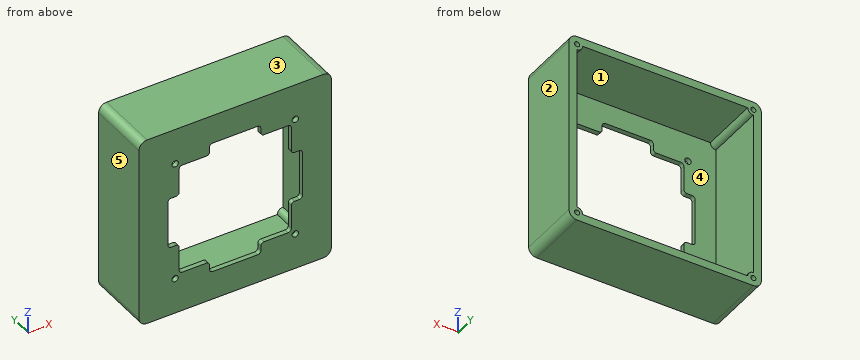
Autodesk Inventor part; units mm, degrees
ref_plane "YZ Plane" through (0, 0, 0) normal (1, 0, 0) x (0, 1, 0)
ref_plane "XZ Plane" through (0, 0, 0) normal (0, 1, 0) x (-1, 0, 0)
ref_plane "XY Plane" through (0, 0, 0) normal (0, 0, 1) x (1, 0, 0)
sketch "Sketch1" plane through (0, 0, 0) normal (0, 1, 0) x (-1, 0, 0)
  line L0 (-55, 55) -> (55, 55)
  line L1 (55, 55) -> (55, -55)
  line L2 (55, -55) -> (-55, -55)
  line L3 (-55, -55) -> (-55, 55)
  line L4 (-55, 55) -> (55, -55) construction
  line L5 (55, 55) -> (-55, -55) construction
  line L6 (-12.5, 37.5) -> (12.5, 37.5) construction
  line L7 (12.5, 37.5) -> (12.5, -37.5) construction
  line L8 (12.5, -37.5) -> (-12.5, -37.5) construction
  line L9 (-12.5, -37.5) -> (-12.5, 37.5) construction
  line L10 (-12.5, 37.5) -> (12.5, -37.5) construction
  line L11 (12.5, 37.5) -> (-12.5, -37.5) construction
  line L12 (-37.5, 37.5) -> (37.5, 37.5) construction
  line L13 (37.5, 37.5) -> (37.5, -37.5) construction
  line L14 (37.5, -37.5) -> (-37.5, -37.5) construction
  line L15 (-37.5, -37.5) -> (-37.5, 37.5)
  line L16 (-37.5, 37.5) -> (37.5, -37.5) construction
  line L17 (37.5, 37.5) -> (-37.5, -37.5) construction
  circle A0 centre (37.5, -37.5) radius 2
  circle A1 centre (37.5, 37.5) radius 2
  circle A2 centre (-37.5, 37.5) radius 2
  circle A3 centre (-37.5, -37.5) radius 2
  point P0 (0, 0)
  dimension "d0" = 110
  dimension "d1" = 110
  dimension "d2" = 25
  dimension "d3" = 75
  dimension "d4" = 75
  dimension "d5" = 4
  dimension "d6" = 4
  dimension "d7" = 4
  dimension "d8" = 4
extrude "Extrusion1" add sketch "Sketch1" along normal blind 3
sketch "Sketch3" plane through (0, 3, 0) normal (0, 1, 0) x (1, 0, 0)
  line L0 (35, -35) -> (-35, -35)
  line L1 (-35, -35) -> (-35, 35)
  line L2 (-35, 35) -> (35, 35)
  line L3 (35, 35) -> (35, -35)
  line L4 (35, -35) -> (-35, 35) construction
  line L5 (-35, -35) -> (35, 35) construction
  point P0 (0, 0)
  dimension "d18" = 70
  dimension "d19" = 70
extrude "Extrusion3" cut sketch "Sketch3" against normal blind 3
fillet "Fillet1" radius 2 4 edges at (-35, 1.5, 35) (-35, 1.5, -35) (35, 1.5, -35) (35, 1.5, 35)
sketch "Sketch4" plane through (0, 3, 0) normal (0, 1, 0) x (1, 0, 0)
  line L0 (28, -16) -> (42, -16)
  line L1 (42, -16) -> (42, 16)
  line L2 (42, 16) -> (28, 16)
  line L3 (28, 16) -> (28, -16)
  line L4 (28, -16) -> (42, 16) construction
  line L5 (42, -16) -> (28, 16) construction
  line L6 (35, 33) -> (35, -33)
  point P0 (0, 0)
  point P1 (35, 0)
  dimension "d23" = 14
  dimension "d24" = 32
extrude "Extrusion4" cut sketch "Sketch4" against normal blind 3
pattern_circular "Circular Pattern2" count 4 over 360 about axis through (0, 0, 0) along (0, 1, 0) of "Extrusion4"
fillet "Fillet2" radius 2 16 edges at (16, 1.5, 35) (-16, 1.5, 35) (16, 1.5, 42) (-16, 1.5, 42) (-35, 1.5, 16) (-42, 1.5, 16) (-42, 1.5, -16) (-35, 1.5, -16) (-16, 1.5, -35) (-16, 1.5, -42) (16, 1.5, -42) (16, 1.5, -35) (35, 1.5, -16) (42, 1.5, -16) (42, 1.5, 16) (35, 1.5, 16)
sketch "Sketch5" plane through (0, 0, 0) normal (0, -1, 0) x (1, 0, 0)
  line L0 (55, -55) -> (-55, -55)
  line L1 (-55, 55) -> (55, 55)
  line L2 (55, 55) -> (55, -55)
  line L3 (55, -55) -> (-55, -55)
  line L4 (-55, -55) -> (-55, 55)
  line L5 (-55, 55) -> (55, -55) construction
  line L6 (55, 55) -> (-55, -55) construction
  line L7 (-60, 60) -> (60, 60)
  line L8 (60, 60) -> (60, -60)
  line L9 (60, -60) -> (-60, -60)
  line L10 (-60, -60) -> (-60, 60)
  line L11 (-60, 60) -> (60, -60) construction
  line L12 (60, 60) -> (-60, -60) construction
  point P0 (0, 0)
  dimension "d31" = 5
extrude "Extrusion5" add sketch "Sketch5" against normal blind 40
sketch "Sketch6" plane through (0, 40, 0) normal (0, 1, 0) x (1, 0, 0)
  line L0 (-55, -55) -> (55, -55)
  circle A0 centre (-55, -55) radius 3.5
  line L1 (-55, -55) -> (-55, 55)
  circle A1 centre (-55, 55) radius 3.5
  line L2 (55, 55) -> (55, -55)
  circle A2 centre (55, 55) radius 3.5
  circle A3 centre (55, -55) radius 3.5
  point P0 (0, 0)
  dimension "d34" = 7
  dimension "d35" = 7
  dimension "d36" = 7
  dimension "d37" = 7
extrude "Extrusion6" add sketch "Sketch6" against normal up to surface (37 mm away)
sketch "Sketch7" plane through (0, 40, 0) normal (0, 1, 0) x (1, 0, 0)
  arc A0 (55, -51.5) -> (51.5, -55) centre (55, -55) ccw
  circle A1 centre (55, -55) radius 1.6
  arc A2 (51.5, 55) -> (55, 51.5) centre (55, 55) ccw
  circle A3 centre (55, 55) radius 1.6
  arc A4 (-55, 51.5) -> (-51.5, 55) centre (-55, 55) ccw
  circle A5 centre (-55, 55) radius 1.6
  arc A6 (-51.5, -55) -> (-55, -51.5) centre (-55, -55) ccw
  circle A7 centre (-55, -55) radius 1.6
  point P0 (0, 0)
  dimension "d40" = 3.2
  dimension "d41" = 3.2
  dimension "d42" = 3.2
  dimension "d43" = 3.2
extrude "Extrusion7" cut sketch "Sketch7" against normal blind 4.5
fillet "Fillet3" radius 5 4 edges at (60, 20, -60) (-60, 20, -60) (60, 20, 60) (-60, 20, 60)
properties part number "3D printed box"
Design review of the part built by this model. Coordinates are the model's own, in mm. Face numbers are marked on the shaded views. A direction names the side the tool comes from. Round coordinates to 2 decimals unless told otherwise and drop trailing zeros. Loops run counter-clockwise (first coordinate to the right, second up) from the corner with the lowest first, then second, coordinate; pieces in that order, holes last. Notation, with made-up numbers: (26.5, 18) -> (42.5, 18) arc R20 ccw to (42.5, 54) -> close; hole circle Ø2 at (-36.75, -11.5). An arc over 180 degrees is marked (long way). Use one line per item in the form item = value. Start each with the question number.
Q1. We need section B-B on y = 7. Give the boundary of the cut face in (x, z), then the cut area to 3 significant figures.
Q2. Draft analysis for pull direction Z (two halves, no side actions). For the marked faces 3, 4 and 5, state which applies: +Z half, -Z half, draft (parallel to the pull), parting line (faces both ways), or undercut.
Q3. We need section C-C on z = 47. Give the boundary of the cut face in (x, y), then the cut area to 3 significant figures.
Q4. We need section A-A on x = -0.5. Give the boundary of the cut face in (y, z).
Q5. For pin 1 Ø1 at (x, z) = (55, -54.5) entering from +Y; pin 2 Ø5 at (x, z) = (-20.5, 43) entering from +Y, all flat-tipped, find the tip position at first contact; note any pin that passes through.
Q6. Wall thickness on line 1 along Z through (x, y) = (37.5, 1.75); line 2 along Z through (x, y) = (-41, 4): over which ranges is each line inside the solid? List them lowest first. Write a range as [from, to].
Q7. We need section D-D on x = -30. Give the boundary of the cut face in (y, z), then the cut area to 3 significant figures.
Q8. Machinability: for the marked faces 1 and 2, which of the approach directions +Z, -Z, +X, -X, +Y, -Y give a long, thin tool a straight path to every point of the face, cutting with its end or side? Answer none if there is none.
Calculated:
q1.outline = (-60, -55) arc R5 ccw to (-55, -60) -> (55, -60) arc R5 ccw to (60, -55) -> (60, 55) arc R5 ccw to (55, 60) -> (-55, 60) arc R5 ccw to (-60, 55) -> close; hole (-55, -51.5) arc R3.5 cw to (-51.5, -55) -> (51.5, -55) arc R3.5 cw to (55, -51.5) -> (55, 51.5) arc R3.5 cw to (51.5, 55) -> (-51.5, 55) arc R3.5 cw to (-55, 51.5) -> close
q1.area = 2,320 mm²
q2.face_3 = +Z half
q2.face_4 = undercut
q2.face_5 = draft
q3.outline = (-60, 0) -> (60, 0) -> (60, 40) -> (55, 40) -> (55, 3) -> (-55, 3) -> (-55, 40) -> (-60, 40) -> close
q3.area = 730 mm²
q4.outline = (0, -60) -> (40, -60) -> (40, -55) -> (3, -55) -> (3, -42) -> (0, -42) -> close; (0, 42) -> (3, 42) -> (3, 55) -> (40, 55) -> (40, 60) -> (0, 60) -> close
q5.pin_1 = 35.5
q5.pin_2 = 3
q6.line_1 = [-60, -39.5], [-35.5, -16], [16, 35.5], [39.5, 60]
q6.line_2 = [-60, -55], [55, 60]
q7.outline = (0, -60) -> (40, -60) -> (40, -55) -> (3, -55) -> (3, -35) -> (0, -35) -> close; (0, 35) -> (3, 35) -> (3, 55) -> (40, 55) -> (40, 60) -> (0, 60) -> close
q7.area = 520 mm²
q8.face_1 = +Y
q8.face_2 = +Z, -Z, +X, +Y, -Y
